Build history of the part. All positions in model axes, mm. Round coordinates to 2 decimals unless told otherwise and drop trailing zeros. Order: outer loops, then holes, each group sorted by start corner. A loop starts at its lowest first (then second) coordinate and runs counter-clockwise, first axis right, second up. Notation, with made-up numbers: M -22,7 L -4,7 A21 ccw -4,28 Z; hole C 33,55.25 d3. An arc over 180 degrees is marked long. Use CSV: the item, a comma, the result in double quotes.
from build123d import *

# Parameters (mm, degrees)
SKETCH_1_W                     = 40
SKETCH_1_H                     = 66.7
EXTRUDE_1_DEPTH                = 2
SKETCH_2_W                     = 4
SKETCH_2_H                     = 66.7
EXTRUDE_2_DEPTH                = 100
CUT_EXTRUDE_1_DEPTH            = 115.526077816
CUT_EXTRUDE_1_DEPTH_BACK       = 115.526077816
HOLE_WIZARD_M4_1_D             = 3.3
HOLE_WIZARD_M4_1_CSINK_D       = 4.05
HOLE_WIZARD_M4_1_CSINK_ANGLE   = 90
HOLE_WIZARD_M4_2_AT_2_COUNT    = 2
HOLE_WIZARD_M4_2_AT_2_PITCH    = 68.59294731
HOLE_WIZARD_M4_2_AT_3_COUNT    = 2
HOLE_WIZARD_M4_2_AT_3_PITCH    = 26
HOLE_WIZARD_M4_2_AT_4_COUNT    = 2
HOLE_WIZARD_M4_2_AT_4_PITCH    = 62.376998966
HOLE_WIZARD_M4_2_AT_5_COUNT    = 2
HOLE_WIZARD_M4_2_AT_5_PITCH    = 56.7
SKETCH_11_W                    = 66.7
SKETCH_11_H                    = 2
EXTRUDE_3_DEPTH                = 100
SKETCH_13_W                    = 40
SKETCH_13_H                    = 66.7
EXTRUDE_4_DEPTH                = 2
SKETCH_14_W                    = 4
SKETCH_14_H                    = 66.7
EXTRUDE_5_DEPTH                = 100
CUT_EXTRUDE_2_DEPTH            = 180.589037806
CUT_EXTRUDE_2_DEPTH_BACK       = 180.589037806
HOLE_WIZARD_M4_3_AT_2_COUNT    = 2
HOLE_WIZARD_M4_3_AT_2_PITCH    = 26
HOLE_WIZARD_M4_3_AT_3_COUNT    = 2
HOLE_WIZARD_M4_3_AT_3_PITCH    = 62.376998966
HOLE_WIZARD_M4_3_AT_4_COUNT    = 2
HOLE_WIZARD_M4_3_AT_4_PITCH    = 56.7
CUT_EXTRUDE_3_REACH            = 181.589
SKETCH_18_R                    = 9.5
CUT_EXTRUDE_4_REACH            = 181.589
SKETCH_21_R                    = 11
CUT_EXTRUDE_5_REACH            = 181.589
SKETCH_22_R                    = 4.5
FILLET_1_R                     = 2
CUT_EXTRUDE_6_REACH            = 193.604
SKETCH_23_W                    = 36
SKETCH_23_H                    = 66.7
CUT_EXTRUDE_7_REACH            = 164.752
SKETCH_24_W                    = 36
SKETCH_24_H                    = 66.7
HOLE_WIZARD_M3_1_D             = 2.5
HOLE_WIZARD_M3_1_CSINK_D       = 3.05
HOLE_WIZARD_M3_1_CSINK_ANGLE   = 90
CUT_EXTRUDE_8_DEPTH            = 154.990981879
CUT_EXTRUDE_8_DEPTH_BACK       = 154.990981879
SKETCH_27_W                    = 4
SKETCH_27_H                    = 66.7
HOLE_WIZARD_M2_5_1_D           = 2.05
HOLE_WIZARD_M2_5_1_CSINK_D     = 2.55
HOLE_WIZARD_M2_5_1_CSINK_ANGLE = 90
FILLET_2_R                     = 0.8


with BuildPart() as part:
    # Sketch 1 → Extrude 1 (new body)
    with BuildSketch(Plane(origin=(0, 0, 0), x_dir=(1, 0, 0), z_dir=(0, 1, 0))):
        Rectangle(SKETCH_1_W, SKETCH_1_H)
    extrude(amount=EXTRUDE_1_DEPTH)

    # Sketch 2 → Extrude 2 (add)
    with BuildSketch(Plane(origin=(0, 2, 0), x_dir=(1, 0, 0), z_dir=(0, 1, 0))):
        with Locations((-18, 0)):
            Rectangle(SKETCH_2_W, SKETCH_2_H)
    extrude(amount=EXTRUDE_2_DEPTH)

    # Sketch 5 → Cut-Extrude 1 (cut, two sides: drawn at the far end of the back side and taken through both)
    with BuildSketch(Plane.ZY.offset(20).offset(-CUT_EXTRUDE_1_DEPTH_BACK)):
        with BuildLine():
            ThreePointArc((0, 102), (23.582011153, 92.232011153), (33.35, 68.65))
            Line((33.35, 68.65), (33.35, 102))
            Line((33.35, 102), (0, 102))
        make_face()
        with BuildLine():
            ThreePointArc((-33.35, 68.65), (-23.582011153, 92.232011153), (0, 102))
            Line((0, 102), (-33.35, 102))
            Line((-33.35, 102), (-33.35, 68.65))
        make_face()
    extrude(amount=CUT_EXTRUDE_1_DEPTH + CUT_EXTRUDE_1_DEPTH_BACK, mode=Mode.SUBTRACT)

    # Hole Wizard M4 _1 (through all)
    with Locations(Plane.ZY.offset(20)):
        with Locations((0, 97.65), (25.11473671, 54.15), (-25.11473671, 54.15)):
            CounterSinkHole(HOLE_WIZARD_M4_1_D / 2, HOLE_WIZARD_M4_1_CSINK_D / 2, counter_sink_angle=HOLE_WIZARD_M4_1_CSINK_ANGLE)

    # Sketch 10 → Hole Wizard M4 _2 (revolve, cut)
    with BuildSketch(Plane(origin=(15, 2, -28.35), x_dir=(0, 0, 1), z_dir=(1, 0, 0))):
        Polygon((0, 0), (0, 2), (1.65, 2), (1.65, 0.375), (2.025, 0), align=None)
    hole_wizard_m4_2 = revolve(axis=Axis((15, 8.35, -28.35), (0, -1, 0)), mode=Mode.SUBTRACT)

    # Hole Wizard M4 _2 at 2: Hole Wizard M4 _2 ×2
    with Locations(*[Vector(-0.9508085645250022, 0, 0.3097790722852413) * (i * HOLE_WIZARD_M4_2_AT_2_PITCH) for i in range(1, HOLE_WIZARD_M4_2_AT_2_COUNT)]):
        add(hole_wizard_m4_2, mode=Mode.SUBTRACT)

    # Hole Wizard M4 _2 at 3: Hole Wizard M4 _2 ×2
    with Locations(*[(-i * HOLE_WIZARD_M4_2_AT_3_PITCH, 0, 0) for i in range(1, HOLE_WIZARD_M4_2_AT_3_COUNT)]):
        add(hole_wizard_m4_2, mode=Mode.SUBTRACT)

    # Hole Wizard M4 _2 at 4: Hole Wizard M4 _2 ×2
    with Locations(*[Vector(-0.4168203092647413, 0, 0.9089889052042635) * (i * HOLE_WIZARD_M4_2_AT_4_PITCH) for i in range(1, HOLE_WIZARD_M4_2_AT_4_COUNT)]):
        add(hole_wizard_m4_2, mode=Mode.SUBTRACT)

    # Hole Wizard M4 _2 at 5: Hole Wizard M4 _2 ×2
    with Locations(*[(0, 0, i * HOLE_WIZARD_M4_2_AT_5_PITCH) for i in range(1, HOLE_WIZARD_M4_2_AT_5_COUNT)]):
        add(hole_wizard_m4_2, mode=Mode.SUBTRACT)

    # Sketch 11 → Extrude 3 (add)
    with BuildSketch(Plane.ZY.offset(20)):
        with Locations((0, 16)):
            Rectangle(SKETCH_11_W, SKETCH_11_H)
    extrude(amount=EXTRUDE_3_DEPTH)



with BuildPart() as body_2:
    # Sketch 13 → Extrude 4 (new body)
    with BuildSketch(Plane(origin=(0, 0, 0), x_dir=(1, 0, 0), z_dir=(0, 1, 0))):
        with Locations((-140, 0)):
            Rectangle(SKETCH_13_W, SKETCH_13_H)
    extrude(amount=EXTRUDE_4_DEPTH)


with BuildPart() as part_1:
    add(part.part)

    add(body_2.part)  # Extrude 5 merges body 2
    # Sketch 14 → Extrude 5 (add)
    with BuildSketch(Plane(origin=(0, 2, 0), x_dir=(1, 0, 0), z_dir=(0, 1, 0))):
        with Locations((-122, 0)):
            Rectangle(SKETCH_14_W, SKETCH_14_H)
    extrude(amount=EXTRUDE_5_DEPTH)

    # Sketch 15 → Cut-Extrude 2 (cut, two sides: drawn at the far end of the back side and taken through both)
    with BuildSketch(Plane.ZY.offset(124).offset(-CUT_EXTRUDE_2_DEPTH_BACK)):
        with BuildLine():
            ThreePointArc((0, 102), (23.582011153, 92.232011153), (33.35, 68.65))
            Line((33.35, 68.65), (33.35, 102))
            Line((33.35, 102), (0, 102))
        make_face()
        with BuildLine():
            ThreePointArc((-33.35, 68.65), (-23.582011153, 92.232011153), (0, 102))
            Line((0, 102), (-33.35, 102))
            Line((-33.35, 102), (-33.35, 68.65))
        make_face()
    extrude(amount=CUT_EXTRUDE_2_DEPTH + CUT_EXTRUDE_2_DEPTH_BACK, mode=Mode.SUBTRACT)

    # Sketch 17 → Hole Wizard M4 _3 (revolve, cut)
    with BuildSketch(Plane(origin=(-129, 2, -28.35), x_dir=(0, 0, 1), z_dir=(1, 0, 0))):
        Polygon((0, 0), (0, 2), (1.65, 2), (1.65, 0.375), (2.025, 0), align=None)
    hole_wizard_m4_3 = revolve(axis=Axis((-129, 8.35, -28.35), (0, -1, 0)), mode=Mode.SUBTRACT)

    # Hole Wizard M4 _3 at 2: Hole Wizard M4 _3 ×2
    with Locations(*[(-i * HOLE_WIZARD_M4_3_AT_2_PITCH, 0, 0) for i in range(1, HOLE_WIZARD_M4_3_AT_2_COUNT)]):
        add(hole_wizard_m4_3, mode=Mode.SUBTRACT)

    # Hole Wizard M4 _3 at 3: Hole Wizard M4 _3 ×2
    with Locations(*[Vector(-0.41682030926474106, 0, 0.9089889052042636) * (i * HOLE_WIZARD_M4_3_AT_3_PITCH) for i in range(1, HOLE_WIZARD_M4_3_AT_3_COUNT)]):
        add(hole_wizard_m4_3, mode=Mode.SUBTRACT)

    # Hole Wizard M4 _3 at 4: Hole Wizard M4 _3 ×2
    with Locations(*[(0, 0, i * HOLE_WIZARD_M4_3_AT_4_PITCH) for i in range(1, HOLE_WIZARD_M4_3_AT_4_COUNT)]):
        add(hole_wizard_m4_3, mode=Mode.SUBTRACT)

    # Sketch 18 → Cut-Extrude 3 (cut, up to next)
    with BuildSketch(Plane.ZY.offset(124), mode=Mode.PRIVATE) as cut_extrude_3_sk1:
        with Locations((0, 68.65)):
            Circle(SKETCH_18_R)
    cut_extrude_3_tool1 = extrude(cut_extrude_3_sk1.sketch, amount=-CUT_EXTRUDE_3_REACH, mode=Mode.PRIVATE) & part_1.part
    add(cut_extrude_3_tool1.solids().sort_by_distance((-124, 68.65, 0))[0], mode=Mode.SUBTRACT)

    # Sketch 21 → Cut-Extrude 4 (cut, up to next)
    with BuildSketch(Plane(origin=(-16, 0, 0), x_dir=(0, 0, -1), z_dir=(1, 0, 0)), mode=Mode.PRIVATE) as cut_extrude_4_sk1:
        with Locations((0, 68.65)):
            Circle(SKETCH_21_R)
    cut_extrude_4_tool1 = extrude(cut_extrude_4_sk1.sketch, amount=-CUT_EXTRUDE_4_REACH, mode=Mode.PRIVATE) & part_1.part
    add(cut_extrude_4_tool1.solids().sort_by_distance((-16, 68.65, 0))[0], mode=Mode.SUBTRACT)

    # Sketch 22 → Cut-Extrude 5 (cut, up to next)
    with BuildSketch(Plane(origin=(-16, 0, 0), x_dir=(0, 0, -1), z_dir=(1, 0, 0)), mode=Mode.PRIVATE) as cut_extrude_5_sk1:
        with Locations((16.670989023, 59.025)):
            Circle(SKETCH_22_R)
    cut_extrude_5_tool1 = extrude(cut_extrude_5_sk1.sketch, amount=-CUT_EXTRUDE_5_REACH, mode=Mode.PRIVATE) & part_1.part
    add(cut_extrude_5_tool1.solids().sort_by_distance((-16, 59.025, -16.670989))[0], mode=Mode.SUBTRACT)

    # Fillet 1
    fillet_1_edges = [part_1.edges().sort_by_distance(p)[0] for p in [
        (-160, 1, -33.35),
        (-160, 1, 33.35),
        (20, 1, 33.35),
        (20, 1, -33.35),
    ]]
    fillet(fillet_1_edges, radius=FILLET_1_R)

    # Sketch 23 → Cut-Extrude 6 (cut, up to next)
    with BuildSketch(Plane(origin=(0, 2, 0), x_dir=(1, 0, 0), z_dir=(0, 1, 0)), mode=Mode.PRIVATE) as cut_extrude_6_sk1:
        with Locations((-142, 0)):
            Rectangle(SKETCH_23_W, SKETCH_23_H)
    cut_extrude_6_tool1 = extrude(cut_extrude_6_sk1.sketch, amount=-CUT_EXTRUDE_6_REACH, mode=Mode.PRIVATE) & part_1.part
    add(cut_extrude_6_tool1.solids().sort_by_distance((-142, 2, 0))[0], mode=Mode.SUBTRACT)

    # Sketch 24 → Cut-Extrude 7 (cut, up to next)
    with BuildSketch(Plane(origin=(0, 2, 0), x_dir=(1, 0, 0), z_dir=(0, 1, 0)), mode=Mode.PRIVATE) as cut_extrude_7_sk1:
        with Locations((2, 0)):
            Rectangle(SKETCH_24_W, SKETCH_24_H)
    cut_extrude_7_tool1 = extrude(cut_extrude_7_sk1.sketch, amount=-CUT_EXTRUDE_7_REACH, mode=Mode.PRIVATE) & part_1.part
    add(cut_extrude_7_tool1.solids().sort_by_distance((2, 2, 0))[0], mode=Mode.SUBTRACT)

    # Hole Wizard M3 _1 (through all)
    with Locations(Plane(origin=(-16, 0, 0), x_dir=(0, 0, -1), z_dir=(1, 0, 0))):
        with Locations((9, 6), (-9, 6)):
            CounterSinkHole(HOLE_WIZARD_M3_1_D / 2, HOLE_WIZARD_M3_1_CSINK_D / 2, counter_sink_angle=HOLE_WIZARD_M3_1_CSINK_ANGLE)

    # Sketch 27 → Cut-Extrude 8 (cut, two sides: drawn at the far end of the back side and taken through both)
    with BuildSketch(Plane(origin=(0, 17, 0), x_dir=(1, 0, 0), z_dir=(0, 1, 0)).offset(-CUT_EXTRUDE_8_DEPTH_BACK)):
        with Locations((-122, 0)):
            Rectangle(SKETCH_27_W, SKETCH_27_H)
        with Locations((-18, 0)):
            Rectangle(SKETCH_27_W, SKETCH_27_H)
    extrude(amount=CUT_EXTRUDE_8_DEPTH + CUT_EXTRUDE_8_DEPTH_BACK, mode=Mode.SUBTRACT)

    # Hole Wizard M2.5 _1 (through all)
    with Locations(Plane(origin=(0, 17, 0), x_dir=(1, 0, 0), z_dir=(0, 1, 0))):
        with Locations((-116, 4), (-116, -4), (-24, 4), (-24, -4)):
            CounterSinkHole(HOLE_WIZARD_M2_5_1_D / 2, HOLE_WIZARD_M2_5_1_CSINK_D / 2, counter_sink_angle=HOLE_WIZARD_M2_5_1_CSINK_ANGLE)

    # Fillet 2
    fillet_2_edges = [part_1.edges().sort_by_distance(p)[0] for p in [
        (-70, 17, -33.35),
        (-20, 15, 0),
        (-70, 15, -33.35),
        (-70, 15, 33.35),
        (-120, 17, 0),
        (-70, 17, 33.35),
        (-120, 15, 0),
        (-20, 17, 0),
        (-120, 16, -33.35),
        (-120, 16, 33.35),
        (-20, 16, -33.35),
        (-20, 16, 33.35),
    ]]
    fillet(fillet_2_edges, radius=FILLET_2_R)


solid = part_1.part
(1) Drop flat-ended pins along their axis: pin 1 (1.8 mm diameter, centred on x = -116, z = -4, fed in from -Y); pin 2 (2.5 mm diameter, centred on x = -116, z = 4, fed in from +Y) (3 decimals). Give the stop position or say it passes through.
Answer block:
pin 1,"passes through"
pin 2,"stops at y = 16.975"
(2) Two-plate mould, pull along X, no slides. Class faces 1 (the face through (-69, 17, 0)), 2 (the face through (-116.978, 15.863, -4.308)): released by +X, released by -X, zero draft, split by the parting line, or undercut.
Answer block:
face 1,"zero draft"
face 2,"undercut"
(3) Wall check: line 1 (Z direction, x = -24, y = 15.95) (3 decimals); line 2 (Z direction, x = -24, y = 15.7) (3 decimals); line 3 (X direction, y = 16.2, z = 4) (3 decimals). Give the ranges that are in metal, low to high. Write a range as from..to.
Answer block:
line 1,"z = -33.35..-5.025, -2.975..2.975, 5.025..33.35"
line 2,"z = -33.344..-5.025, -2.975..2.975, 5.025..33.344"
line 3,"x = -120..-117.025, -114.975..-25.025, -22.975..-20"
(4) Cut at A-A, the plane x = -116. Give the cut face in (y, z) (3 decimals).
Answer block:
outline,"M 15,-32.55 A0.8 ccw 15.8,-33.35 L 16.2,-33.35 A0.8 ccw 17,-32.55 L 17,-5.275 L 16.75,-5.025 L 15,-5.025 Z; M 15,-2.975 L 16.75,-2.975 L 17,-2.725 L 17,2.725 L 16.75,2.975 L 15,2.975 Z; M 15,5.025 L 16.75,5.025 L 17,5.275 L 17,32.55 A0.8 ccw 16.2,33.35 L 15.8,33.35 A0.8 ccw 15,32.55 Z"
(5) Cut at B-B, the plane z = -4. Give the cut face in (x, y) (3 decimals).
Answer block:
outline,"M -120,15.8 A0.8 ccw -119.2,15 L -117.025,15 L -117.025,16.75 L -117.275,17 L -119.2,17 A0.8 ccw -120,16.2 Z; M -114.975,15 L -25.025,15 L -25.025,16.75 L -25.275,17 L -114.725,17 L -114.975,16.75 Z; M -22.975,15 L -20.8,15 A0.8 ccw -20,15.8 L -20,16.2 A0.8 ccw -20.8,17 L -22.725,17 L -22.975,16.75 Z"
